from build123d import *

# Parameters (mm, degrees)
SKETCH_3_W          = 9.5
SKETCH_3_H          = 16.1
CUT_EXTRUDE_1_DEPTH = 80.130651457
SKETCH_4_R          = 4
CUT_EXTRUDE_2_DEPTH = 6
SKETCH_5_R          = 10
CUT_EXTRUDE_3_DEPTH = 50
SKETCH_6_R          = 7
CUT_EXTRUDE_4_DEPTH = 30
SKETCH_7_R          = 3
CUT_EXTRUDE_5_DEPTH = 45.4


with BuildPart() as part:
    # 草图1 → 旋转1 (revolve)
    with BuildSketch(Plane(origin=(0, 0, 0), x_dir=(1, 0, 0), z_dir=(0, 1, 0))):
        Polygon((0, -65.4), (12.6875, -65.4), (22.225, 0), (31.5, 0), (31.5, 15.9), (20, 15.9), (20, 59), (19, 60), (0, 60), align=None)
    revolve(axis=Axis((0, 0, 65.4), (0, 0, -1)))

    # 草图2 → 切除-旋转1 (revolve, cut)
    with BuildSketch(Plane(origin=(0, 0, 0), x_dir=(1, 0, 0), z_dir=(0, 1, 0))):
        Polygon((28, 8), (32, 5.6906), (32, 10.3094), align=None)
    revolve(axis=Axis((0, 0, 0), (0, 0, 1)), mode=Mode.SUBTRACT)

    # 草图3 → 切除-拉伸1 (cut, through all)
    with BuildSketch(Plane.XY):
        with Locations((28.25, 0)):
            Rectangle(SKETCH_3_W, SKETCH_3_H)
        with Locations((-28.25, 0)):
            Rectangle(SKETCH_3_W, SKETCH_3_H)
    extrude(amount=-CUT_EXTRUDE_1_DEPTH, mode=Mode.SUBTRACT)

    # 草图4 → 切除-拉伸2 (cut)
    with BuildSketch(Plane.XY.offset(-15.9)):
        with Locations((0, 25)):
            Circle(SKETCH_4_R)
    extrude(amount=CUT_EXTRUDE_2_DEPTH, mode=Mode.SUBTRACT)

    # 草图5 → 切除-拉伸3 (cut)
    with BuildSketch(Plane.XY.offset(-60)):
        Circle(SKETCH_5_R)
    extrude(amount=CUT_EXTRUDE_3_DEPTH, mode=Mode.SUBTRACT)

    # 草图6 → 切除-拉伸4 (cut)
    with BuildSketch(Plane.XY.offset(65.4)):
        Circle(SKETCH_6_R)
    extrude(amount=-CUT_EXTRUDE_4_DEPTH, mode=Mode.SUBTRACT)

    # 草图7 → 切除-拉伸5 (cut)
    with BuildSketch(Plane.XY.offset(-10)):
        Circle(SKETCH_7_R)
    extrude(amount=CUT_EXTRUDE_5_DEPTH, mode=Mode.SUBTRACT)


solid = part.part
Part model, mm, in its own coordinate system. A direction names the side the tool comes from. Coordinates: 2 decimals unless noted, no trailing zeros. Order: outer loops, then holes, each group sorted by start corner. A loop starts at its lowest first (then second) coordinate and runs counter-clockwise, first axis right, second up.
(1) Pull direction X, two halves, no side cores. Call faces 1 (the face through (-0.579, 31.495, -3.031)), 2 (the face through (-3, 0, 12)), 3 (the face through (-5.5, 5.5, 65.4)): pulls with the +X half, pulls with the -X half, needs draft (parallel to the pull), parting line crosses it, or undercut.
Check sheet entries:
face 1: parting line crosses it
face 2: undercut
face 3: needs draft
(2) Tool access for faces 4 (the face through (-22.4, -2.5, 0)), 5 (the face through (0.579, -31.495, -3.031)), 6 (the face through (-4.336, 19.524, -37.752)), 7 (the face through (-23.5, 0, -8)): list every direction of +Z, -Z, +X, -X, +Y, -Y with a clear straight run to the whole face (end or side of a thin tool).
Check sheet entries:
face 4: +Z
face 5: +Z, -Z, -Y
face 6: -Z
face 7: +Z, -Z, -X
(3) Slice it at A-A, the plane z = -2.5. Write the cut outline in (x, y).
Check sheet entries:
outline: (-30.45, -8.05) arc R31.5 ccw to (30.45, -8.05) - (23.5, -8.05) - (23.5, 8.05) - (30.45, 8.05) arc R31.5 ccw to (-30.45, 8.05) - (-23.5, 8.05) - (-23.5, -8.05) - close; hole circle Ø6 at (0, 0)
(4) Pin check, flat tips, straight feed: pin 1 Ø1.5 at (x, y) = (-11.5, 22) entering from -Z; pin 2 Ø8 at (y, z) = (-2.5, -5) entering from +X; pin 3 Ø3 at (x, z) = (9, -5) entering from +Y; pin 4 Ø3.5 at (x, y) = (0, 0) entering from +Z. Stop position of each tip, or through.
Check sheet entries:
pin 1: stops at z = -15.9
pin 2: stops at x = 23.5
pin 3: stops at y = 30.59
pin 4: passes through
(5) Slice it at D-D, the plane z = 18.5. Write the cut outline in (x, y).
Check sheet entries:
outline: circle Ø39.05 at (0, 0); hole circle Ø6 at (0, 0)
(6) Slice it at C-C, the plane z = -20. Write the cut outline in (x, y).
Check sheet entries:
outline: circle Ø40 at (0, 0); hole circle Ø20 at (0, 0)
(7) Slice it at B-B, the plane y = 0. Write the cut outline in (x, z) (1 decimal), and give its area (3 significant figures).
Check sheet entries:
outline: (-23.5, -15.9) - (-20, -15.9) - (-20, -59) - (-19, -60) - (-10, -60) - (-10, -10) - (-3, -10) - (-3, 35.4) - (-7, 35.4) - (-7, 65.4) - (-12.7, 65.4) - (-22.2, 0) - (-23.5, 0) - close; (3, -10) - (10, -10) - (10, -60) - (19, -60) - (20, -59) - (20, -15.9) - (23.5, -15.9) - (23.5, 0) - (22.2, 0) - (12.7, 65.4) - (7, 65.4) - (7, 35.4) - (3, 35.4) - close
area: 3,100 mm2
(8) Probe L1, parallel to Y at x = 0, z = -34.5; L2, parallel to Z at x = 8, y = 2; L3, parallel to Y at x = 0, z = 51. List the from-to ranges inside material, lowest first.
Check sheet entries:
L1: y = -20 to -10, 10 to 20
L2: z = -10 to 65.4
L3: y = -14.79 to -7, 7 to 14.79
